Check sheet for the modelled part. Datum: model origin and axes. Units: mm. A direction names the side the tool comes from. Round coordinates to 2 decimals unless told otherwise and drop trailing zeros. Loops run counter-clockwise (first coordinate to the right, second up) from the corner with the lowest first, then second, coordinate; pieces in that order, holes last. Notation, with made-up numbers: (40, 24) -> (83, 24) arc R17 cw to (83, 39) -> close; hole circle Ø1 at (1.25, 5). An arc over 180 degrees is marked (long way). One line per question, with ' | ' between items.
```python
from build123d import *

# Parameters (mm, degrees)
SKETCH1_W                      = 676.28516
SKETCH1_H                      = 310.642
BASE_FLANGE1_DEPTH             = 3.175
EDGE_FLANGE2_STRIP_W           = 19.05
EDGE_FLANGE2_STRIP_H           = 3.175
EDGE_FLANGE2_STRIP_CUT_DEPTH   = 310.642
EDGE_FLANGE2_STRIP_2_W         = 19.05
EDGE_FLANGE2_STRIP_2_H         = 3.175
EDGE_FLANGE2_STRIP_CUT_2_DEPTH = 310.642
EDGE_FLANGE2_DEPTH             = 310.642
EDGE_FLANGE2_BEND_DEPTH        = 310.642
EDGE_FLANGE3_DEPTH             = 676.28516
EDGE_FLANGE3_2_DEPTH           = 6.35
EDGE_FLANGE3_START             = 669.93516
EDGE_FLANGE3_3_DEPTH           = 6.35
EDGE_FLANGE3_START_2           = 6.35
EDGE_FLANGE3_4_DEPTH           = 663.58516


# Read off the part's stored shape, not the designer's step: Edge-Flange3
# Sheet-metal steps are written as plain solids
with BuildPart() as part:
    # Sketch1 → Base-Flange1 (new body)
    with BuildSketch(Plane(origin=(0, 0, 0), x_dir=(1, 0, 0), z_dir=(0, 1, 0))):
        with Locations((338.14258, 155.321)):
            Rectangle(SKETCH1_W, SKETCH1_H)
    extrude(amount=-BASE_FLANGE1_DEPTH)

    # Edge-Flange2 strip (across the edge) → Edge-Flange2 strip cut (cut)
    with BuildSketch(Plane(origin=(676.28516, 0, 0), x_dir=(-1, 0, 0), z_dir=(0, 0, -1))):
        with Locations((-3.175, -1.5875)):
            Rectangle(EDGE_FLANGE2_STRIP_W, EDGE_FLANGE2_STRIP_H)
    extrude(amount=EDGE_FLANGE2_STRIP_CUT_DEPTH, mode=Mode.SUBTRACT)

    # Edge-Flange2 strip 2 (across the edge) → Edge-Flange2 strip cut 2 (cut)
    with BuildSketch(Plane.XY.offset(-310.642)):
        with Locations((-3.175, -1.5875)):
            Rectangle(EDGE_FLANGE2_STRIP_2_W, EDGE_FLANGE2_STRIP_2_H)
    extrude(amount=EDGE_FLANGE2_STRIP_CUT_2_DEPTH, mode=Mode.SUBTRACT)

    # Edge-Flange2 section (across the edge) → Edge-Flange2 (add)
    with BuildSketch(Plane(origin=(676.28516, 0, 0), x_dir=(-1, 0, 0), z_dir=(0, 0, -1))):
        with BuildLine():
            Line((0, 3.175), (0, 22.225))
            Line((0, 22.225), (3.175, 22.225))
            Line((3.175, 22.225), (3.175, 3.175))
            ThreePointArc((3.175, 3.175), (4.10493597, 0.92993597), (6.35, 0))
            Line((6.35, 0), (6.35, -3.175))
            ThreePointArc((6.35, -3.175), (1.859871939, -1.315128061), (0, 3.175))
        make_face()
    extrude(amount=EDGE_FLANGE2_DEPTH)

    # Edge-Flange2 section 2 (across the edge) → Edge-Flange2 bend (add)
    with BuildSketch(Plane.XY.offset(-310.642)):
        with BuildLine():
            Line((0, 3.175), (0, 22.225))
            Line((0, 22.225), (3.175, 22.225))
            Line((3.175, 22.225), (3.175, 3.175))
            ThreePointArc((3.175, 3.175), (4.10493597, 0.92993597), (6.35, 0))
            Line((6.35, 0), (6.35, -3.175))
            ThreePointArc((6.35, -3.175), (1.859871939, -1.315128061), (0, 3.175))
        make_face()
    extrude(amount=EDGE_FLANGE2_BEND_DEPTH)

    # Edge-Flange3 outline → Edge-Flange3 (cut)
    with BuildSketch(Plane.YZ):
        with BuildLine():
            Line((3.175, -310.642), (3.175, -307.467))
            Line((3.175, -307.467), (0, -307.467))
            ThreePointArc((0, -307.467), (0.92993597, -309.71206403), (3.175, -310.642))
        make_face()
        with BuildLine():
            ThreePointArc((-2.324261315, -310.642), (-2.958628997, -309.110500936), (-3.175, -307.467))
            Line((-3.175, -307.467), (-3.175, -310.642))
            Line((-3.175, -310.642), (-2.324261315, -310.642))
        make_face()
    extrude(amount=EDGE_FLANGE3_DEPTH, mode=Mode.SUBTRACT)

    # Edge-Flange3 2 outline → Edge-Flange3 2 (cut)
    with BuildSketch(Plane.YZ):
        with BuildLine():
            ThreePointArc((3.175, -310.642), (0.92993597, -309.71206403), (0, -307.467))
            Line((0, -307.467), (-3.175, -307.467))
            ThreePointArc((-3.175, -307.467), (-2.958628997, -309.110500936), (-2.324261315, -310.642))
            Line((-2.324261315, -310.642), (3.175, -310.642))
        make_face()
    extrude(amount=EDGE_FLANGE3_2_DEPTH, mode=Mode.SUBTRACT)

    # Edge-Flange3 3 outline → Edge-Flange3 3 (cut)
    with BuildSketch(Plane.YZ.offset(EDGE_FLANGE3_START)):
        with BuildLine():
            ThreePointArc((3.175, -310.642), (0.92993597, -309.71206403), (0, -307.467))
            Line((0, -307.467), (-3.175, -307.467))
            ThreePointArc((-3.175, -307.467), (-2.958628997, -309.110500936), (-2.324261315, -310.642))
            Line((-2.324261315, -310.642), (3.175, -310.642))
        make_face()
    extrude(amount=EDGE_FLANGE3_3_DEPTH, mode=Mode.SUBTRACT)

    # Edge-Flange3 4 outline → Edge-Flange3 4 (add)
    with BuildSketch(Plane.YZ.offset(EDGE_FLANGE3_START_2)):
        with BuildLine():
            Line((0, -307.467), (0, -310.642))
            Line((0, -310.642), (-2.324261315, -310.642))
            ThreePointArc((-2.324261315, -310.642), (-1e-09, -312.966261314), (3.175, -313.817))
            Line((3.175, -313.817), (22.225, -313.817))
            Line((22.225, -313.817), (22.225, -310.642))
            Line((22.225, -310.642), (3.175, -310.642))
            ThreePointArc((3.175, -310.642), (0.92993597, -309.71206403), (0, -307.467))
        make_face()
    extrude(amount=EDGE_FLANGE3_4_DEPTH)


solid = part.part
```
(1) Scan lines: probe 1 along X at (y, z) = (20, -56.5) (3 decimals); probe 2 along Y at (x, z) = (591, -160) (3 decimals); probe 3 along Z at (x, y) = (384, 16.5). Record each from-to range of solid material in increasing order.
Answer:
probe 1: x = 0 to 3.175, 673.11 to 676.285 | probe 2: y = -3.175 to 0 | probe 3: z = -313.82 to -310.64
(2) Mould release check, pull along X, two halves, no side actions. Record for faces 4 (the face through (3.175, 13, -157)), 5 (the face through (676.285, 13, -153)), 6 (the face through (333, -3.175, -156)): +X half, -X half, draft (parallel to the pull), parting line (faces both ways), or undercut.
Answer:
face 4: undercut | face 5: +X half | face 6: draft
(3) Set-up check for faces 1 (the face through (333, 13, -310.642)), 2 (the face through (673.11, 13, -153)), 3 (the face through (0, 13, -157)): record each of +Z, -Z, +X, -X, +Y, -Y from which the full face is reachable in a straight line by a thin tool's end or side.
Answer:
face 1: +Z, +Y | face 2: +Z, -Z, +Y | face 3: +Z, -Z, -X, +Y, -Y
(4) Sectioned sample at C-C, the plane x = 250.5. Record the cut outline in (y, z) (3 decimals), and give its area (3 significant figures).
Answer:
outline: (-3.175, -307.467) arc R6.35 ccw to (3.175, -313.817) -> (22.225, -313.817) -> (22.225, -310.642) -> (3.175, -310.642) arc R3.175 cw to (0, -307.467) -> (0, 0) -> (-3.175, 0) -> close | area: 1,060 mm2
(5) Sectioned sample at A-A, the plane y = 8. Record the cut outline in (x, z) (3 decimals).
Answer:
outline: (0, -310.642) -> (3.175, -310.642) -> (3.175, 0) -> (0, 0) -> close; (6.35, -313.817) -> (669.935, -313.817) -> (669.935, -310.642) -> (6.35, -310.642) -> close; (673.11, -310.642) -> (676.285, -310.642) -> (676.285, 0) -> (673.11, 0) -> close
(6) Sectioned sample at B-B, the plane z = -293.5. Record the cut outline in (x, y) (3 decimals).
Answer:
outline: (0, 3.175) arc R6.35 ccw to (6.35, -3.175) -> (669.935, -3.175) arc R6.35 ccw to (676.285, 3.175) -> (676.285, 22.225) -> (673.11, 22.225) -> (673.11, 3.175) arc R3.175 cw to (669.935, 0) -> (6.35, 0) arc R3.175 cw to (3.175, 3.175) -> (3.175, 22.225) -> (0, 22.225) -> close
(7) Go/stop test with flat-tipped pins: pin 1 (1 mm diameter, centred on x = 180, y = 8, fed in from +Z); pin 2 (2.5 mm diameter, centred on x = 675.5, y = 15.5, fed in from -Z); pin 3 (10 mm diameter, centred on x = 238.5, z = -273.5, fed in from +Y). Record where each tip stops, or that it passes through.
Answer:
pin 1: stops at z = -310.64 | pin 2: stops at z = -310.64 | pin 3: stops at y = 0
